```python
from build123d import *

# Parameters (mm, degrees)
SKETCH_1_R          = 30
EXTRUDE_3_DEPTH     = 6
SKETCH_6_R          = 25
CUT_EXTRUDE_1_DEPTH = 2
CUT_EXTRUDE_START   = 4
SKETCH_4_R          = 25
CUT_EXTRUDE_2_DEPTH = 2
SKETCH_8_R          = 6
EXTRUDE_5_DEPTH     = 10
SKETCH_10_R         = 2
CUT_EXTRUDE_6_DEPTH = 10


with BuildPart() as part:
    # 草图1 → 凸台-拉伸3 (new body)
    with BuildSketch(Plane(origin=(0, 0, 0), x_dir=(1, 0, 0), z_dir=(0, 1, 0))):
        with Locations(Location((0, 0, 0), (0, 0, 270))):
            Circle(SKETCH_1_R)
    extrude(amount=EXTRUDE_3_DEPTH)

    # 草图6 → 切除-拉伸1 (cut)
    with BuildSketch(Plane.XZ):
        with Locations(Location((0, 0, 0), (0, 0, 270))):
            Circle(SKETCH_6_R)
    extrude(amount=-CUT_EXTRUDE_1_DEPTH, mode=Mode.SUBTRACT)

    # 草图4 → 切除-拉伸2 (cut)
    with BuildSketch(Plane(origin=(0, 0, 0), x_dir=(1, 0, 0), z_dir=(0, 1, 0)).offset(CUT_EXTRUDE_START)):
        with Locations(Location((0, 0, 0), (0, 0, 90))):
            Circle(SKETCH_4_R)
    extrude(amount=CUT_EXTRUDE_2_DEPTH, mode=Mode.SUBTRACT)

    # 草图8 → 凸台-拉伸5 (add)
    with BuildSketch(Plane(origin=(0, 2, 0), x_dir=(-1, 0, 0), z_dir=(0, -1, 0))):
        with Locations(Location((0, 0, 0), (0, 0, 90))):
            Circle(SKETCH_8_R)
    extrude(amount=EXTRUDE_5_DEPTH)

    # 草图10 → 切除-拉伸6 (cut)
    with BuildSketch(Plane(origin=(0, -8, 0), x_dir=(-1, 0, 0), z_dir=(0, -1, 0))):
        with Locations(Location((0, 0, 0), (0, 0, 90))):
            Circle(SKETCH_10_R)
    extrude(amount=-CUT_EXTRUDE_6_DEPTH, mode=Mode.SUBTRACT)


solid = part.part
```
Could you check a few things on this model? Use its own coordinates, in mm. A direction names the side the tool comes from. Round coordinates to 2 decimals unless told otherwise and drop trailing zeros. Order: outer loops, then holes, each group sorted by start corner. A loop starts at its lowest first (then second) coordinate and runs counter-clockwise, first axis right, second up. Notation, with made-up numbers: M 29.25,5 L 57.25,5 A13 cw 57.25,28 Z; hole C -34,-28 d9. An arc over 180 degrees is marked long. One line per question, with ' | ' between items. Start each with the question number.
(1) Suppose I cut it at A-A on z = 0. List the corners of the cut face in (x, y) for me.
(2) For faces 1 (the face through (0, 4, 0)), 2 (the face through (25, 6, -7)), 3 (the face through (-2, -3, 0)), which set-ups out of +Z, -Z, +X, -X, +Y, -Y let a thin tool reach every point of the face, with its end or its side?
(3) For P1, Ø2, axis at x = -6, y = -5.5, coming from the +Z side; P2, Ø8, axis at x = -3, z = -20.5, coming from the +Y side; P3, Ø1.5, axis at x = -19.5, y = 1.5, coming from the +Z side; P4, Ø4.5, axis at x = 0, z = 0, coming from the -Y side, each with a flat end and sliding along its axis, tell me the tip position at first contact or that it passes through.
(4) Suppose I cut it at B-B on x = 0. List the corners of the cut face in (y, z) for me, then the cut area to 3 significant figures.
(5) Thinking about a two-plate mould opening in X: for faces 4 (the face through (25, 0, -7)), 5 (the face through (-7.509, 4.986, -23.846)), 6 (the face through (1.802, -2.93, -5.723)), 7 (the face through (1.32, 2.96, -29.97)), which applies, +X half, -X half, draft (parallel to the pull), parting line (faces both ways), or undercut?
(6) Suppose I cut it at C-C on y = -3.5. List the corners of the cut face in (x, z) for me, then the cut area to 3 significant figures.
(7) Please list where these lines run through material, in increasing order: line 1 along X through (y, z) = (1.15, 0); line 2 along X through (y, z) = (-4.75, 0); line 3 along Z through (x, y) = (-0.5, 0.25) (1 decimal).
(8) Suppose I cut it at D-D on x = 14.5. List the corners of the cut face in (y, z) for me.
Geometry results:
1) outline: M -30,0 L -25,0 L -25,2 L -6,2 L -6,-8 L -2,-8 L -2,2 L 2,2 L 2,-8 L 6,-8 L 6,2 L 25,2 L 25,0 L 30,0 L 30,6 L 25,6 L 25,4 L -25,4 L -25,6 L -30,6 Z
2) face 1: +Y | face 2: +Z, -Z, +X, -X, +Y | face 3: -Y
3) P1: z = 3.32 | P2: y = 4 | P3: z = 23.42 | P4: y = -8
4) outline: M -8,-6 L 2,-6 L 2,-25 L 0,-25 L 0,-30 L 6,-30 L 6,-25 L 4,-25 L 4,25 L 6,25 L 6,30 L 0,30 L 0,25 L 2,25 L 2,6 L -8,6 L -8,2 L 2,2 L 2,-2 L -8,-2 Z | area: 240 mm²
5) face 4: draft | face 5: undercut | face 6: undercut | face 7: parting line
6) outline: C 0,0 d12; hole C 0,0 d4 | area: 101 mm²
7) line 1: -30 to -25, -6 to -2, 2 to 6, 25 to 30 | line 2: -6 to -2, 2 to 6 | line 3: -30 to -25, -6 to -1.9, 1.9 to 6, 25 to 30
8) outline: M 0,-26.26 L 6,-26.26 L 6,-20.37 L 4,-20.37 L 4,20.37 L 6,20.37 L 6,26.26 L 0,26.26 L 0,20.37 L 2,20.37 L 2,-20.37 L 0,-20.37 Z
